Verification items for the finished model (mm, model axes). A direction names the side the tool comes from. Coordinates: 2 decimals unless noted, no trailing zeros. Order: outer loops, then holes, each group sorted by start corner. A loop starts at its lowest first (then second) coordinate and runs counter-clockwise, first axis right, second up. Notation, with made-up numbers: (23, 52) - (47, 52) arc R17 cw to (47, 73) - close; hole circle Ø5 at (40.25, -3). An arc over 180 degrees is marked (long way). Answer as CSV lines item,"result". Start each with the question number.
1. Section check A-A (y = -23.5). Record the cut outline in (x, z), and give its area (3 significant figures).
2. Material ranges on L1, parallel to X at y = -36.5, z = 0; L2, parallel to Z at x = -82.55, y = -35.5; L3, parallel to Z at x = 101.6, y = -32, recorded low to high. Write a range as [from, to].
3. Go/stop test with a flat-tipped pin: pin 1 (9 mm diameter, centred on y = 41.275, z = 0, fed in from +X) (3 decimals). Record where the tip stops, or that it passes through.
4. Mould release check, pull along Z, two halves, no side actions. Record for faces 4 (the cylindrical face through (-2.472, -32.964, -4.754)), 5 (the conical face through (66.914, 41.932, 0.207)), 6 (the flat face through (-2, -1, -12.7)), 7 (the flat face through (120.65, -1, 0)): pulls with the +Z half, pulls with the -Z half, needs draft (parallel to the pull), parting line crosses it, or undercut.
5. Set-up check for faces 1 (the flat face through (95.885, 38, -3)), 2 (the cylindrical face through (-96.247, -32.964, 0.236)), 3 (the flat face through (-120.65, -1, 0)): record each of +Z, -Z, +X, -X, +Y, -Y from which the full face is reachable in a straight line by a thin tool's end or side.
from build123d import *

# Parameters (mm, degrees)
F0_W     = 241.3
F0_H     = 25.4
F1_DEPTH = 50.8
F2_R     = 6.35
F3_DEPTH = 24.765
F5_D     = 7.9375
F5_DEPTH = 27.0002
F5_TIP   = 2.3846655818
F7_D     = 10.71626
F7_DEPTH = 35.179
F7_TIP   = 3.2194893086
F8_D     = 12.7
F8_DEPTH = 38.1
F8_TIP   = 3.8154649308


# Not quite as in the source:
# - a length typed as a fraction of an inch, garbled in the dataset ("3 / 203.2 mm" for 3/8 in), is restored


with BuildPart() as f1:
    # F0 (on Front) → F1 (new body, symmetric)
    with BuildSketch(Plane.XZ):
        Rectangle(F0_W, F0_H)
    extrude(amount=F1_DEPTH, both=True)

    # F2 (on face) → F3 (cut)
    with BuildSketch(Plane.YZ.offset(120.65)):
        with Locations((41.275, 0)):
            Circle(F2_R)
    extrude(amount=-F3_DEPTH, mode=Mode.SUBTRACT)

    # F5
    with Locations(Plane.YZ.offset(95.885)):
        with Locations((41.275, 0)):
            Hole(F5_D / 2, depth=F5_DEPTH)
            with Locations((0, 0, -(F5_DEPTH + F5_TIP / 2))):  # 118° drill point
                Cone(0, F5_D / 2, F5_TIP, mode=Mode.SUBTRACT)

    # F7
    with Locations(Plane.XZ.offset(50.8)):
        with Locations((-101.6, 0), (0, 0), (101.6, 0)):
            Hole(F7_D / 2, depth=F7_DEPTH)
            with Locations((0, 0, -(F7_DEPTH + F7_TIP / 2))):  # 118° drill point
                Cone(0, F7_D / 2, F7_TIP, mode=Mode.SUBTRACT)

    # F8
    with Locations(Plane.XZ.offset(50.8)):
        with Locations((-82.55, 0), (82.55, 0)):
            Hole(F8_D / 2, depth=F8_DEPTH)
            with Locations((0, 0, -(F8_DEPTH + F8_TIP / 2))):  # 118° drill point
                Cone(0, F8_D / 2, F8_TIP, mode=Mode.SUBTRACT)


solid = f1.part
Evaluation:
1,outline,"(-120.65, -12.7) - (120.65, -12.7) - (120.65, 12.7) - (-120.65, 12.7) - close; hole circle Ø10.72 at (-101.6, 0); hole circle Ø12.7 at (-82.55, 0); hole circle Ø10.72 at (0, 0); hole circle Ø12.7 at (82.55, 0); hole circle Ø10.72 at (101.6, 0)"
1,area,"5,610 mm²"
2,L1,"x = [-120.65, -106.96], [-96.24, -88.9], [-76.2, -5.36], [5.36, 76.2], [88.9, 96.24], [106.96, 120.65]"
2,L2,"z = [-12.7, -6.35], [6.35, 12.7]"
2,L3,"z = [-12.7, -5.36], [5.36, 12.7]"
3,pin 1,"stops at x = 95.885"
4,face 4,"undercut"
4,face 5,"undercut"
4,face 6,"pulls with the -Z half"
4,face 7,"needs draft"
5,face 1,"+X"
5,face 2,"-Y"
5,face 3,"+Z, -Z, -X, +Y, -Y"
